Check sheet for the modelled part. Datum: model origin and axes. Units: mm. Face numbers are marked on the shaded views. A direction names the side the tool comes from. Give positions to 0.01 mm unless a question says otherwise; leave off trailing zeros. Order: outer loops, then holes, each group sorted by start corner. A loop starts at its lowest first (then second) coordinate and runs counter-clockwise, first axis right, second up.
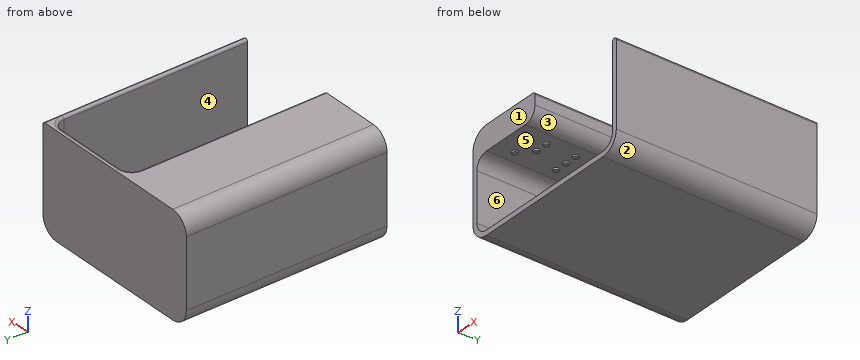
from build123d import *
from OCP.BRepFilletAPI import BRepFilletAPI_MakeChamfer

# Parameters (mm, degrees)
BOSS_EXTRUDE1_DEPTH = 80
SKETCH2_W           = 74
SKETCH2_H           = 42
BOSS_EXTRUDE2_DEPTH = 2
FILLET1_R           = 5
FILLET2_R           = 7
FILLET3_R           = 5
FILLET5_R           = 1
SKETCH3_R           = 1
BOSS_EXTRUDE4_DEPTH = 0.5
CHAMFER1_SIZE       = 0.288675135
CHAMFER1_SIZE_2     = 0.5


with BuildPart() as part:
    # Sketch1 → Boss-Extrude1 (new body)
    with BuildSketch(Plane(origin=(0, 0, 0), x_dir=(1, 0, 0), z_dir=(0, 1, 0))):
        Polygon((0, 0), (74, 0), (74, -42), (72, -42), (72, -2), (2, -2), (2, -32), (32, -32), (32, -42), (0, -42), align=None)
    extrude(amount=BOSS_EXTRUDE1_DEPTH)

    # Sketch2 → Boss-Extrude2 (add)
    with BuildSketch(Plane(origin=(0, 80, 0), x_dir=(1, 0, 0), z_dir=(0, 1, 0))):
        with Locations((37, -21)):
            Rectangle(SKETCH2_W, SKETCH2_H)
    extrude(amount=BOSS_EXTRUDE2_DEPTH)

    # Fillet1
    fillet1_edges = [part.edges().sort_by_distance(p)[0] for p in [
        (72, 40, 2),
        (2, 40, 2),
        (2, 40, 32),
        (32, 40, 32),
    ]]
    fillet(fillet1_edges, radius=FILLET1_R)

    # Fillet2
    fillet2_edges = [part.edges().sort_by_distance(p)[0] for p in [
        (0, 41, 0),
        (74, 41, 0),
        (0, 41, 42),
    ]]
    fillet(fillet2_edges, radius=FILLET2_R)

    # Fillet3
    fillet3_edges = [part.edges().sort_by_distance(p)[0] for p in [
        (32, 80, 39.5),
        (17, 80, 32),
        (2, 80, 17),
        (37, 80, 2),
        (72, 80, 24.5),
        (3.464466094, 80, 3.464466094),
        (70.535533906, 80, 3.464466094),
        (3.464466094, 80, 30.535533906),
        (30.535533906, 80, 33.464466094),
    ]]
    fillet(fillet3_edges, radius=FILLET3_R)

    # Fillet5
    fillet5_edges = [part.edges().sort_by_distance(p)[0] for p in [
        (70.535533906, 78.535533906, 42),
        (74, 41, 42),
        (52, 80, 42),
        (32, 37.5, 42),
        (72, 37.5, 42),
        (33.464466094, 78.535533906, 42),
    ]]
    fillet(fillet5_edges, radius=FILLET5_R - 0.0001)  # a hair under: the kernel refuses the full size

    # Sketch3 → Boss-Extrude4 (add)
    with BuildSketch(Plane(origin=(0, 0, 32), x_dir=(-1, 0, 0), z_dir=(0, 0, -1))):
        with Locations(Location((-12, 72.5, 0), (0, 0, 180))):
            Circle(SKETCH3_R)
        with Locations(Location((-12, 67.5, 0), (0, 0, 180))):
            Circle(SKETCH3_R)
        with Locations(Location((-12, 60.5, 0), (0, 0, 180))):
            Circle(SKETCH3_R)
        with Locations(Location((-12, 48.5, 0), (0, 0, 180))):
            Circle(SKETCH3_R)
        with Locations(Location((-17, 43.5, 0), (0, 0, 180))):
            Circle(SKETCH3_R)
        with Locations(Location((-17, 48.5, 0), (0, 0, 180))):
            Circle(SKETCH3_R)
        with Locations(Location((-22, 48.5, 0), (0, 0, 180))):
            Circle(SKETCH3_R)
        with Locations(Location((-12, 36.5, 0), (0, 0, 180))):
            Circle(SKETCH3_R)
        with Locations(Location((-17, 31.5, 0), (0, 0, 180))):
            Circle(SKETCH3_R)
        with Locations(Location((-22, 36.5, 0), (0, 0, 180))):
            Circle(SKETCH3_R)
        with Locations(Location((-12, 24.5, 0), (0, 0, 180))):
            Circle(SKETCH3_R)
        with Locations(Location((-17, 24.5, 0), (0, 0, 180))):
            Circle(SKETCH3_R)
        with Locations(Location((-22, 24.5, 0), (0, 0, 180))):
            Circle(SKETCH3_R)
        with Locations(Location((-22, 12.5, 0), (0, 0, 180))):
            Circle(SKETCH3_R)
        with Locations(Location((-17, 12.5, 0), (0, 0, 180))):
            Circle(SKETCH3_R)
        with Locations(Location((-12, 7.5, 0), (0, 0, 180))):
            Circle(SKETCH3_R)
    extrude(amount=BOSS_EXTRUDE4_DEPTH)

    # Chamfer1
    chamfer1_edges_1 = [part.edges().sort_by_distance(p)[0] for p in [
        (11, 67.5, 32),
    ]]
    chamfer1_side_1 = [part.faces().sort_by_distance(p)[0] for p in [
        (10.994226497, 67.5, 32),
    ]]
    chamfer1_edges_2 = [part.edges().sort_by_distance(p)[0] for p in [
        (11, 60.5, 32),
    ]]
    chamfer1_side_2 = [part.faces().sort_by_distance(p)[0] for p in [
        (10.994226497, 60.5, 32),
    ]]
    chamfer1_edges_3 = [part.edges().sort_by_distance(p)[0] for p in [
        (11, 48.5, 32),
    ]]
    chamfer1_side_3 = [part.faces().sort_by_distance(p)[0] for p in [
        (10.994226497, 48.5, 32),
    ]]
    chamfer1_edges_4 = [part.edges().sort_by_distance(p)[0] for p in [
        (11, 72.5, 32),
    ]]
    chamfer1_side_4 = [part.faces().sort_by_distance(p)[0] for p in [
        (10.994226497, 72.5, 32),
    ]]
    chamfer1_edges_5 = [part.edges().sort_by_distance(p)[0] for p in [
        (16, 43.5, 32),
    ]]
    chamfer1_side_5 = [part.faces().sort_by_distance(p)[0] for p in [
        (15.994226497, 43.5, 32),
    ]]
    chamfer1_edges_6 = [part.edges().sort_by_distance(p)[0] for p in [
        (16, 48.5, 32),
    ]]
    chamfer1_side_6 = [part.faces().sort_by_distance(p)[0] for p in [
        (15.994226497, 48.5, 32),
    ]]
    chamfer1_edges_7 = [part.edges().sort_by_distance(p)[0] for p in [
        (21, 48.5, 32),
    ]]
    chamfer1_side_7 = [part.faces().sort_by_distance(p)[0] for p in [
        (20.994226497, 48.5, 32),
    ]]
    chamfer1_edges_8 = [part.edges().sort_by_distance(p)[0] for p in [
        (11, 36.5, 32),
    ]]
    chamfer1_side_8 = [part.faces().sort_by_distance(p)[0] for p in [
        (10.994226497, 36.5, 32),
    ]]
    chamfer1_edges_9 = [part.edges().sort_by_distance(p)[0] for p in [
        (16, 31.5, 32),
    ]]
    chamfer1_side_9 = [part.faces().sort_by_distance(p)[0] for p in [
        (15.994226497, 31.5, 32),
    ]]
    chamfer1_edges_10 = [part.edges().sort_by_distance(p)[0] for p in [
        (21, 36.5, 32),
    ]]
    chamfer1_side_10 = [part.faces().sort_by_distance(p)[0] for p in [
        (20.994226497, 36.5, 32),
    ]]
    chamfer1_edges_11 = [part.edges().sort_by_distance(p)[0] for p in [
        (11, 24.5, 32),
    ]]
    chamfer1_side_11 = [part.faces().sort_by_distance(p)[0] for p in [
        (10.994226497, 24.5, 32),
    ]]
    chamfer1_edges_12 = [part.edges().sort_by_distance(p)[0] for p in [
        (16, 24.5, 32),
    ]]
    chamfer1_side_12 = [part.faces().sort_by_distance(p)[0] for p in [
        (15.994226497, 24.5, 32),
    ]]
    chamfer1_edges_13 = [part.edges().sort_by_distance(p)[0] for p in [
        (21, 24.5, 32),
    ]]
    chamfer1_side_13 = [part.faces().sort_by_distance(p)[0] for p in [
        (20.994226497, 24.5, 32),
    ]]
    chamfer1_edges_14 = [part.edges().sort_by_distance(p)[0] for p in [
        (21, 12.5, 32),
    ]]
    chamfer1_side_14 = [part.faces().sort_by_distance(p)[0] for p in [
        (20.994226497, 12.5, 32),
    ]]
    chamfer1_edges_15 = [part.edges().sort_by_distance(p)[0] for p in [
        (16, 12.5, 32),
    ]]
    chamfer1_side_15 = [part.faces().sort_by_distance(p)[0] for p in [
        (15.994226497, 12.5, 32),
    ]]
    chamfer1_edges_16 = [part.edges().sort_by_distance(p)[0] for p in [
        (11, 7.5, 32),
    ]]
    chamfer1_side_16 = [part.faces().sort_by_distance(p)[0] for p in [
        (10.994226497, 7.5, 32),
    ]]
    chamfer1 = BRepFilletAPI_MakeChamfer(part.part.solid().wrapped)
    for e in chamfer1_edges_1:
        chamfer1.Add(CHAMFER1_SIZE - 0.0001, CHAMFER1_SIZE_2 - 0.0001, e.wrapped, chamfer1_side_1[0].wrapped)
    for e in chamfer1_edges_2:
        chamfer1.Add(CHAMFER1_SIZE - 0.0001, CHAMFER1_SIZE_2 - 0.0001, e.wrapped, chamfer1_side_2[0].wrapped)
    for e in chamfer1_edges_3:
        chamfer1.Add(CHAMFER1_SIZE - 0.0001, CHAMFER1_SIZE_2 - 0.0001, e.wrapped, chamfer1_side_3[0].wrapped)
    for e in chamfer1_edges_4:
        chamfer1.Add(CHAMFER1_SIZE - 0.0001, CHAMFER1_SIZE_2 - 0.0001, e.wrapped, chamfer1_side_4[0].wrapped)
    for e in chamfer1_edges_5:
        chamfer1.Add(CHAMFER1_SIZE - 0.0001, CHAMFER1_SIZE_2 - 0.0001, e.wrapped, chamfer1_side_5[0].wrapped)
    for e in chamfer1_edges_6:
        chamfer1.Add(CHAMFER1_SIZE - 0.0001, CHAMFER1_SIZE_2 - 0.0001, e.wrapped, chamfer1_side_6[0].wrapped)
    for e in chamfer1_edges_7:
        chamfer1.Add(CHAMFER1_SIZE - 0.0001, CHAMFER1_SIZE_2 - 0.0001, e.wrapped, chamfer1_side_7[0].wrapped)
    for e in chamfer1_edges_8:
        chamfer1.Add(CHAMFER1_SIZE - 0.0001, CHAMFER1_SIZE_2 - 0.0001, e.wrapped, chamfer1_side_8[0].wrapped)
    for e in chamfer1_edges_9:
        chamfer1.Add(CHAMFER1_SIZE - 0.0001, CHAMFER1_SIZE_2 - 0.0001, e.wrapped, chamfer1_side_9[0].wrapped)
    for e in chamfer1_edges_10:
        chamfer1.Add(CHAMFER1_SIZE - 0.0001, CHAMFER1_SIZE_2 - 0.0001, e.wrapped, chamfer1_side_10[0].wrapped)
    for e in chamfer1_edges_11:
        chamfer1.Add(CHAMFER1_SIZE - 0.0001, CHAMFER1_SIZE_2 - 0.0001, e.wrapped, chamfer1_side_11[0].wrapped)
    for e in chamfer1_edges_12:
        chamfer1.Add(CHAMFER1_SIZE - 0.0001, CHAMFER1_SIZE_2 - 0.0001, e.wrapped, chamfer1_side_12[0].wrapped)
    for e in chamfer1_edges_13:
        chamfer1.Add(CHAMFER1_SIZE - 0.0001, CHAMFER1_SIZE_2 - 0.0001, e.wrapped, chamfer1_side_13[0].wrapped)
    for e in chamfer1_edges_14:
        chamfer1.Add(CHAMFER1_SIZE - 0.0001, CHAMFER1_SIZE_2 - 0.0001, e.wrapped, chamfer1_side_14[0].wrapped)
    for e in chamfer1_edges_15:
        chamfer1.Add(CHAMFER1_SIZE - 0.0001, CHAMFER1_SIZE_2 - 0.0001, e.wrapped, chamfer1_side_15[0].wrapped)
    for e in chamfer1_edges_16:
        chamfer1.Add(CHAMFER1_SIZE - 0.0001, CHAMFER1_SIZE_2 - 0.0001, e.wrapped, chamfer1_side_16[0].wrapped)
    add(Compound.cast(chamfer1.Shape()), mode=Mode.REPLACE)  # a hair under: the kernel refuses the full size


solid = part.part
1) Depth check by flat-ended pin: pin 1 Ø2 at (x, z) = (20.5, 8.5) entering from -Y; pin 2 Ø8 at (x, y) = (59, 47.5) entering from +Z. Enter the tip coordinate at first touch or a pass-through.
Recorded:
pin 1: stops at y = 80
pin 2: stops at z = 2
2) Material ranges on L1, parallel to Z at x = 24, y = 50.5; L2, parallel to X at y = 43.5, z = 19; L3, parallel to Z at x = 37.5, y = 59.5, recorded low to high.
Recorded:
L1: z = 0 to 2, 32 to 42
L2: x = 0 to 2, 72 to 74
L3: z = 0 to 2
3) Set-up check for the marked faces 4, 5 and 6: record each of +Z, -Z, +X, -X, +Y, -Y from which the full face is reachable in a straight line by a thin tool's end or side.
Recorded:
face 4: +Z, -Y
face 5: none
face 6: -Y
4) Draft check along Z on the marked faces 1, 2 and 3. Enter one of: +Z half, -Z half, draft (parallel to the pull), parting line (faces both ways), or undercut.
Recorded:
face 1: draft
face 2: -Z half
face 3: undercut
5) Section check A-A, the plane x = 66. Record the cut outline in (y, z), then the cut area to 3 significant figures.
Recorded:
outline: (0, 0) - (82, 0) - (82, 42) - (81, 42) arc R1 ccw to (80, 41) - (80, 7) arc R5 cw to (75, 2) - (0, 2) - close
area: 249 mm2
6) Section check C-C, the plane z = 22. Record the cut outline in (x, y).
Recorded:
outline: (0, 0) - (2, 0) - (2, 75) arc R5 cw to (7, 80) - (67, 80) arc R5 cw to (72, 75) - (72, 0) - (74, 0) - (74, 82) - (0, 82) - close
